Source: CAD feature listing. Evaluate the final solid. Frame: model axes, mm. A direction names the side the tool comes from. Give positions to 0.01 mm unless a question says otherwise; leave off trailing zeros. Order: outer loops, then holes, each group sorted by start corner. A loop starts at its lowest first (then second) coordinate and runs counter-clockwise, first axis right, second up. Notation, with made-up numbers: (-2, -25.5) - (55, -25.5) arc R13 ccw to (55, -17.5) - close; hole circle Ø1 at (-35, -4). An arc over 180 degrees is marked (long way). Answer as CSV lines item,"result".
```python
from build123d import *

# Parameters (mm, degrees)
SKETCH_1_R          = 18
EXTRUDE_1_DEPTH     = 92
CUT_EXTRUDE_2_DEPTH = 36
SHELL_8_T           = -1
SKETCH_2_R          = 11
EXTRUDE_2_DEPTH     = 2
SKETCH_3_R          = 4
EXTRUDE_3_DEPTH     = 18
CUT_EXTRUDE_START   = -15
CUT_EXTRUDE_1_DEPTH = 15
SKETCH_5_R          = 5
EXTRUDE_4_DEPTH     = 3
SKETCH_6_R          = 1.5
EXTRUDE_5_DEPTH     = 9
FILLET_1_R          = 1
SKETCH_8_R          = 1.5
CUT_EXTRUDE_3_DEPTH = 5
SKETCH_9_W          = 0.3
SKETCH_9_H          = 9
SKETCH_9_H_2        = 5
EXTRUDE_START       = 1.7
SKETCH_10_R         = 18
EXTRUDE_6_DEPTH     = 1.7
SKETCH_12_R         = 7.5
EXTRUDE_7_DEPTH     = 1.5


with BuildPart() as part:
    # 草图1 → 凸台-拉伸1 (new body)
    with BuildSketch(Plane.XY):
        Circle(SKETCH_1_R)
    extrude(amount=EXTRUDE_1_DEPTH)

    # 草图7 → 切除-拉伸2 (cut)
    with BuildSketch(Plane(origin=(0, 18, 0), x_dir=(1, 0, 0), z_dir=(0, 1, 0))):
        with BuildLine():
            Line((5, -18), (-5, -18))
            ThreePointArc((-5, -18), (-8, -15), (-5, -12))
            Line((-5, -12), (5, -12))
            ThreePointArc((5, -12), (8, -15), (5, -18))
        make_face()
    extrude(amount=-CUT_EXTRUDE_2_DEPTH, mode=Mode.SUBTRACT)

    # 抽壳8
    shell_8_openings = [part.faces().sort_by_distance(p)[0] for p in [
        (8, 0, 15),
        (0, 0, 18),
        (-8, 0, 15),
        (0, 0, 12),
    ]]
    offset(amount=SHELL_8_T, openings=shell_8_openings)

    # 草图2 → 凸台-拉伸2 (add)
    with BuildSketch(Plane.XY.offset(92)):
        Circle(SKETCH_2_R)
    extrude(amount=EXTRUDE_2_DEPTH)

    # 草图3 → 凸台-拉伸3 (add)
    with BuildSketch(Plane.XY.offset(94)):
        Circle(SKETCH_3_R)
    extrude(amount=EXTRUDE_3_DEPTH)

    # 草图4 → 切除-拉伸1 (cut)
    with BuildSketch(Plane.XY.offset(112).offset(CUT_EXTRUDE_START)):
        with BuildLine():
            ThreePointArc((2.645751311, 3), (1.414213562, 3.741657387), (0, 4))
            Line((0, 4), (0, 3))
            Line((0, 3), (2.645751311, 3))
        make_face()
        with BuildLine():
            Line((0, 3), (0, 4))
            ThreePointArc((0, 4), (-1.414213562, 3.741657387), (-2.645751311, 3))
            Line((-2.645751311, 3), (0, 3))
        make_face()
    extrude(amount=CUT_EXTRUDE_1_DEPTH, mode=Mode.SUBTRACT)

    # 草图5 → 凸台-拉伸4 (add)
    with BuildSketch(Plane(origin=(0, 0, 0), x_dir=(-1, 0, 0), z_dir=(0, 0, -1))):
        with Locations(Location((0, 0, 0), (0, 0, 180))):
            Circle(SKETCH_5_R)
    extrude(amount=EXTRUDE_4_DEPTH)

    # 草图6 → 凸台-拉伸5 (add)
    with BuildSketch(Plane(origin=(0, 0, -3), x_dir=(-1, 0, 0), z_dir=(0, 0, -1))):
        Circle(SKETCH_6_R)
    extrude(amount=EXTRUDE_5_DEPTH)

    # 圆角1
    fillet_1_edges = [part.edges().sort_by_distance(p)[0] for p in [
        (1.5, 0, -12),
    ]]
    fillet(fillet_1_edges, radius=FILLET_1_R)

    # 草图8 → 切除-拉伸3 (cut)
    with BuildSketch(Plane.XY.offset(92)):
        with Locations((14, 0)):
            Circle(SKETCH_8_R)
        with Locations((0, -14)):
            Circle(SKETCH_8_R)
        with Locations((-14, 0)):
            Circle(SKETCH_8_R)
        with Locations((0, 14)):
            Circle(SKETCH_8_R)
    extrude(amount=-CUT_EXTRUDE_3_DEPTH, mode=Mode.SUBTRACT)

    # 草图9 → 切除-旋转1 (revolve, cut)
    with BuildSketch(Plane(origin=(0, 0, 0), x_dir=(1, 0, 0), z_dir=(0, 1, 0)), mode=Mode.PRIVATE) as cut_revolve_1_sk:
        with Locations((17.85, -87.5)):
            Rectangle(SKETCH_9_W, SKETCH_9_H)
        with Locations((17.85, -61.5)):
            Rectangle(SKETCH_9_W, SKETCH_9_H_2)
    revolve(cut_revolve_1_sk.sketch.rotate(Axis((0, 0, 0), (0, 0, 1)), 180), axis=Axis((0, 0, 0), (0, 0, 1)), mode=Mode.SUBTRACT)

    # 草图10 → 凸台-拉伸6 (add)
    with BuildSketch(Plane(origin=(0, 0, -3), x_dir=(-1, 0, 0), z_dir=(0, 0, -1)).offset(EXTRUDE_START)):
        Circle(SKETCH_10_R)
    extrude(amount=-EXTRUDE_6_DEPTH)

    # 草图12 → 凸台-拉伸7 (add, symmetric)
    with BuildSketch(Plane(origin=(0, 0, -8.3), x_dir=(-1, 0, 0), z_dir=(0, 0, -1))):
        Circle(SKETCH_12_R)
    extrude(amount=EXTRUDE_7_DEPTH, both=True)


solid = part.part
```
(1) Contact query for flat-ended pins moving along their axis: pin 1 (1.9 mm diameter, centred on x = 1, y = -17, fed in from +Z); pin 2 (1 mm diameter, centred on y = 12, z = 62, fed in from +X); pin 3 (2.5 mm diameter, centred on x = -14, y = 0, fed in from +Z). Output: stop coordinate, or through.
Completed:
pin 1,"z = 92"
pin 2,"x = 13.46"
pin 3,"z = 1"
(2) Cut plane C-C (z = 75). Return loops of the section in (x, y), then the cut area to 3 significant figures.
Completed:
outline,"circle Ø36 at (0, 0); hole circle Ø34 at (0, 0)"
area,"110 mm²"
(3) Access query for faces 1 (the cylindrical face through (1.5, 0.07, -10.39)), 2 (the flat face through (0, 3, 104)), 3 (the flat face through (4, -4, 0)), 4 (the cylindrical face through (-8, 15.9, 15.1)). Directions: +Z, -Z, +X, -X, +Y, -Y. A direction counts if a zero-diameter tool reaches every point of the face in a straight line with its end or side. Return the directions, or none.
Completed:
face 1,"-Z"
face 2,"+Z, +X, -X, +Y"
face 3,"none"
face 4,"+Y, -Y"
(4) Ray query, line 1 (Z direction, x = -13.5, y = -4.5); line 2 (Z direction, x = -1.5, y = 0.5); line 3 (Y direction, x = 0, z = 34). Return the intervals inside material, ascending. Write a range as from..to.
Completed:
line 1,"-4.7..-3, 0..1, 91..92"
line 2,"-9.8..-6.8, -4.7..1, 91..112"
line 3,"-18..-17, 17..18"
(5) Cut plane B-B (x = 14). Return loops of the section in (y, z).
Completed:
outline,"(-11.31, -4.7) - (11.31, -4.7) - (11.31, -3) - (-11.31, -3) - close; (-11.31, 0) - (11.31, 0) - (11.31, 59) - (10.83, 59) - (10.83, 64) - (11.31, 64) - (11.31, 83) - (10.83, 83) - (10.83, 92) - (1.5, 92) - (1.5, 91) - (9.64, 91) - (9.64, 1) - (-9.64, 1) - (-9.64, 91) - (-1.5, 91) - (-1.5, 92) - (-10.83, 92) - (-10.83, 83) - (-11.31, 83) - (-11.31, 64) - (-10.83, 64) - (-10.83, 59) - (-11.31, 59) - close"
(6) Mould query, pull axis X, two halves, no side actions, for faces 5 (the cylindrical face through (-2.38, -10.74, 92.99)), 6 (the cylindrical face through (8, 15.9, 14.9)), 7 (the flat face through (0, -5, 94)). Classes: released by +X, released by -X, zero draft, split by the parting line, or undercut.
Completed:
face 5,"split by the parting line"
face 6,"undercut"
face 7,"zero draft"
(7) Cut plane A-A (y = -9). Return loops of the section in (x, z).
Completed:
outline,"(-15.59, -4.7) - (15.59, -4.7) - (15.59, -3) - (-15.59, -3) - close; (-15.59, 0) - (15.59, 0) - (15.59, 59) - (15.24, 59) - (15.24, 64) - (15.59, 64) - (15.59, 83) - (15.24, 83) - (15.24, 92) - (6.32, 92) - (6.32, 94) - (-6.32, 94) - (-6.32, 92) - (-15.24, 92) - (-15.24, 83) - (-15.59, 83) - (-15.59, 64) - (-15.24, 64) - (-15.24, 59) - (-15.59, 59) - close; hole (-14.42, 1) - (14.42, 1) - (14.42, 91) - (-14.42, 91) - close"
